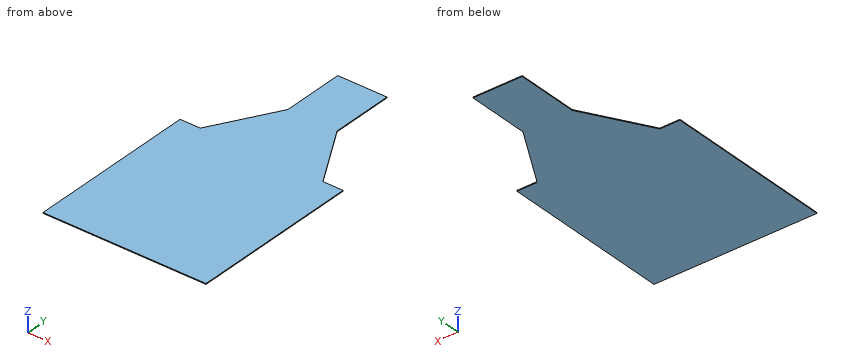
```python
from build123d import *

# Parameters (mm, degrees)
SKETCH2_W          = 400
SKETCH2_H          = 420
BASE_FLANGE1_DEPTH = 2
TAB1_DEPTH         = 2


# Sheet-metal steps are written as plain solids
with BuildPart() as part:
    # Sketch2 → Base-Flange1 (new body)
    with BuildSketch(Plane.XY):
        with Locations((0, 28.575414969)):
            Rectangle(SKETCH2_W, SKETCH2_H)
    extrude(amount=-BASE_FLANGE1_DEPTH)

    # Sketch5 → Tab1 (add)
    with BuildSketch(Plane.XY):
        Polygon((-60.421834446, 394.376455492), (-60.421834446, 547.430628062), (60.421834446, 547.430628062), (60.421834446, 394.376455492), (150.373607132, 238.575414969), (-150.373607132, 238.575414969), align=None)
    extrude(amount=-TAB1_DEPTH)


solid = part.part
```
Build history of the part. All positions in model axes, mm. Give positions to 0.01 mm unless a question says otherwise; leave off trailing zeros. Loops run counter-clockwise (first coordinate to the right, second up) from the corner with the lowest first, then second, coordinate; pieces in that order, holes last.
1) Band-saw the part on B-B on x = 160.5. List the corners of the cut face in (y, z), then the cut area to 3 significant figures.
Values follow:
outline: (-181.42, -2) - (238.58, -2) - (238.58, 0) - (-181.42, 0) - close
area: 840 mm2
2) Drop flat-ended pins along their axis: P1, Ø0.6, axis at y = 475.5, z = -1, coming from the +X side; P2, Ø0.6, axis at y = 465, z = -0.5, coming from the -X side. Give the stop position or say it passes through.
Values follow:
P1: stops at x = 60.42
P2: stops at x = -60.42
3) Band-saw the part on A-A on z = -0.3. List the corners of the cut face in (x, y), then the cut area to 3 significant figures.
Values follow:
outline: (-200, -181.42) - (200, -181.42) - (200, 238.58) - (150.37, 238.58) - (60.42, 394.38) - (60.42, 547.43) - (-60.42, 547.43) - (-60.42, 394.38) - (-150.37, 238.58) - (-200, 238.58) - close
area: 219,000 mm2
4) Probe line 1 along Y through (x, z) = (170, -0.7); line 2 along X through (y, z) = (490.5, -1.85); line 3 along Y through (x, z) = (137, -1.3). List the from-to ranges inside material, lowest first.
Values follow:
line 1: y = -181.42 to 238.58
line 2: x = -60.42 to 60.42
line 3: y = -181.42 to 261.74
5) Band-saw the part on C-C on y = 436. List the corners of the cut face in (x, z).
Values follow:
outline: (-60.42, -2) - (60.42, -2) - (60.42, 0) - (-60.42, 0) - close
